from build123d import *

# Parameters (mm, degrees)
BOSS_EXTRUDE1_DEPTH  = 3.175
M3_CLEARANCE_HOLE1_D = 3.4
SKETCH7_R            = 6.25
CUT_EXTRUDE3_DEPTH   = 92.569651758
FILLET1_R            = 2.5
CHAMFER1_SIZE        = 0.25


with BuildPart() as part:
    # Sketch1 → Boss-Extrude1 (new body)
    with BuildSketch(Plane.XY):
        with BuildLine():
            Line((-53.841624215, 50.764943631), (-53.841624215, 43.491624215))
            Line((-53.841624215, 43.491624215), (-22.5, 43.491624215))
            Line((-22.5, 43.491624215), (-22.5, -43.491624215))
            Line((-22.5, -43.491624215), (-53.841624215, -43.491624215))
            Line((-53.841624215, -43.491624215), (-53.841624215, -50.764943631))
            ThreePointArc((-53.841624215, -50.764943631), (0, -74), (53.841624215, -50.764943631))
            Line((53.841624215, -50.764943631), (53.841624215, -43.491624215))
            Line((53.841624215, -43.491624215), (22.5, -43.491624215))
            Line((22.5, -43.491624215), (22.5, 43.491624215))
            Line((22.5, 43.491624215), (53.841624215, 43.491624215))
            Line((53.841624215, 43.491624215), (53.841624215, 50.764943631))
            ThreePointArc((53.841624215, 50.764943631), (0, 74), (-53.841624215, 50.764943631))
        make_face()
    extrude(amount=BOSS_EXTRUDE1_DEPTH)

    # M3 Clearance Hole1 (through all)
    with Locations(Plane(origin=(48.666624215, 48.666624215, 0), x_dir=(-1, 0, 0), z_dir=(0, 0, -1))):
        with Locations((0, 0), (97.33324843, 0), (97.33324843, -97.33324843), (0, -97.33324843)):
            Hole(M3_CLEARANCE_HOLE1_D / 2)

    # Sketch7 → Cut-Extrude3 (cut, through all)
    with BuildSketch(Plane(origin=(0, 0, 0), x_dir=(-1, 0, 0), z_dir=(0, 0, -1))):
        with Locations((15, 55)):
            Circle(SKETCH7_R)
        with Locations(Location((-15, 55, 0), (0, 0, 180))):
            Circle(SKETCH7_R)
        with Locations((-15, -55)):
            Circle(SKETCH7_R)
        with Locations(Location((15, -55, 0), (0, 0, 180))):
            Circle(SKETCH7_R)
    extrude(amount=-CUT_EXTRUDE3_DEPTH, mode=Mode.SUBTRACT)

    # Fillet1
    fillet1_edges = [part.edges().sort_by_distance(p)[0] for p in [
        (53.841624215, 50.764943631, 1.5875),
        (53.841624215, 43.491624215, 1.5875),
        (22.5, 43.491624215, 1.5875),
        (22.5, -43.491624215, 1.5875),
        (53.841624215, -43.491624215, 1.5875),
        (53.841624215, -50.764943631, 1.5875),
        (-53.841624215, -50.764943631, 1.5875),
        (-53.841624215, -43.491624215, 1.5875),
        (-22.5, -43.491624215, 1.5875),
        (-22.5, 43.491624215, 1.5875),
        (-53.841624215, 43.491624215, 1.5875),
        (-53.841624215, 50.764943631, 1.5875),
    ]]
    fillet(fillet1_edges, radius=FILLET1_R)

    # Chamfer1
    chamfer1_edges = [part.edges().sort_by_distance(p)[0] for p in [
        (23.232233047, 42.759391168, 0),
        (23.232233047, 42.759391168, 3.175),
        (23.232233047, -42.759391168, 0),
        (23.232233047, -42.759391168, 3.175),
        (-23.232233047, -42.759391168, 0),
        (-23.232233047, -42.759391168, 3.175),
        (-23.232233047, 42.759391168, 0),
        (-23.232233047, 42.759391168, 3.175),
        (-21.25, -55, 3.175),
        (-21.25, -55, 0),
        (21.25, -55, 3.175),
        (21.25, -55, 0),
        (8.75, 55, 3.175),
        (8.75, 55, 0),
        (-8.75, 55, 3.175),
        (-8.75, 55, 0),
        (0, 74, 0),
        (0, 74, 3.175),
        (53.841624215, 47.876967743, 0),
        (38.170812108, 43.491624215, 0),
        (22.5, 0, 0),
        (38.170812108, -43.491624215, 0),
        (53.841624215, -47.876967743, 0),
        (0, -74, 0),
        (-53.841624215, -47.876967743, 0),
        (-38.170812108, -43.491624215, 0),
        (-22.5, 0, 0),
        (-38.170812108, 43.491624215, 0),
        (-53.841624215, 47.876967743, 0),
        (-53.65872415, -50.700952785, 0),
        (-53.65872415, 50.700952785, 0),
        (-53.109391168, 44.223857262, 0),
        (-53.109391168, -44.223857262, 0),
        (53.65872415, -50.700952785, 0),
        (53.109391168, -44.223857262, 0),
        (53.109391168, 44.223857262, 0),
        (53.65872415, 50.700952785, 0),
        (53.841624215, 47.876967743, 3.175),
        (-53.841624215, 47.876967743, 3.175),
        (-38.170812108, 43.491624215, 3.175),
        (-22.5, 0, 3.175),
        (-38.170812108, -43.491624215, 3.175),
        (-53.841624215, -47.876967743, 3.175),
        (0, -74, 3.175),
        (53.841624215, -47.876967743, 3.175),
        (38.170812108, -43.491624215, 3.175),
        (22.5, 0, 3.175),
        (38.170812108, 43.491624215, 3.175),
        (-53.65872415, -50.700952785, 3.175),
        (-53.65872415, 50.700952785, 3.175),
        (-53.109391168, 44.223857262, 3.175),
        (-53.109391168, -44.223857262, 3.175),
        (53.65872415, -50.700952785, 3.175),
        (53.109391168, -44.223857262, 3.175),
        (53.109391168, 44.223857262, 3.175),
        (53.65872415, 50.700952785, 3.175),
    ]]
    chamfer(chamfer1_edges, length=CHAMFER1_SIZE)


solid = part.part
Check sheet for the modelled part. Datum: model origin and axes. Units: mm. A direction names the side the tool comes from. Give positions to 0.01 mm unless a question says otherwise; leave off trailing zeros. Order: outer loops, then holes, each group sorted by start corner. A loop starts at its lowest first (then second) coordinate and runs counter-clockwise, first axis right, second up. Notation, with made-up numbers: M -32.75,34 L -21.75,34 A27 cw -21.75,67 Z; hole C 27.25,-12 d6. An arc over 180 degrees is marked long. Answer as CSV lines item,"result". Start each with the question number.
Item 1: Thickness scan on line 1 (X direction, y = -50.5, z = 2.9); line 2 (X direction, y = 54.5, z = 0.95); line 3 (Y direction, x = -15, z = 2.1). Record the ranges inside material, lowest first. Write a range as [from, to].
Item 2: Mould release check, pull along Y, two halves, no side actions. Record for faces 4 (the face through (-1, 1, 0)), 5 (the face through (0.83, 73.995, 1.569)), 6 (the face through (-15.8, -61.2, 1.6)): +Y half, -Y half, draft (parallel to the pull), parting line (faces both ways), or undercut.
Item 3: Gauge pin test, flat ends, axial feed: P1, Ø0.8, axis at x = -38.5, z = 2, coming from the +Y side; P2, Ø1.5, axis at y = -36.5, z = 1, coming from the -X side; P3, Ø1.3, axis at x = 35, z = 2, coming from the -Y side. Record the tip position at first contact, or that the pin passes through.
Item 4: Tool access check on faces 1 (the face through (23.17, 42.87, 0.13)), 2 (the face through (23.125, -42.826, 3.048)), 3 (the face through (-23.125, 42.826, 0.127)). Record the directions out of +Z, -Z, +X, -X, +Y, -Y that give a thin tool (end or side, any length) a straight path to the whole face; none if there is none.
Item 5: Cross-section at B-B on z = 2.2. State how many separate pieces and enclosed holes the cut face has, plus the area to 3 significant figures.
Item 6: Cross-section at A-A on y = -10.5. Enter the section's corners in (x, z) (3 decimals), plus the area to 3 significant figures.
Established:
1,line 1,"x = [-53.73, -19.34], [-10.66, 10.66], [19.34, 53.73]"
1,line 2,"x = [-50.06, -21.23], [-8.77, 8.77], [21.23, 50.06]"
1,line 3,"y = [-72.46, -61.25], [-48.75, 48.75], [61.25, 72.46]"
2,face 4,"draft"
2,face 5,"+Y half"
2,face 6,"undercut"
3,P1,"stops at y = 63.44"
3,P2,"stops at x = -22.5"
3,P3,"stops at y = -65.54"
4,face 1,"-Z, +X"
4,face 2,"+Z, +X"
4,face 3,"-Z, -X"
5,separate pieces,"1"
5,enclosed holes,"8"
5,area,"8,410 mm^2"
6,outline,"M -22.5,0.25 L -22.25,0 L 22.25,0 L 22.5,0.25 L 22.5,2.925 L 22.25,3.175 L -22.25,3.175 L -22.5,2.925 Z"
6,area,"143 mm^2"
